Verification items for the finished model (mm, model axes). A direction names the side the tool comes from. Give positions to 0.01 mm unless a question says otherwise; leave off trailing zeros. Order: outer loops, then holes, each group sorted by start corner. A loop starts at its lowest first (then second) coordinate and runs counter-clockwise, first axis right, second up. Notation, with made-up numbers: (56, 54) - (96, 54) arc R30 cw to (96, 83) - close; hole circle Ø7 at (33.5, 66). An arc over 180 degrees is marked (long way). Answer as a JSON object with one key per item and string values.
Autodesk Inventor part; units mm, degrees
ref_plane "YZ Plane" through (0, 0, 0) normal (1, 0, 0) x (0, 1, 0)
ref_plane "XZ Plane" through (0, 0, 0) normal (0, 1, 0) x (-1, 0, 0)
ref_plane "XY Plane" through (0, 0, 0) normal (0, 0, 1) x (1, 0, 0)
sketch "スケッチ1" plane through (0, 0, 0) normal (1, 0, 0) x (0, 1, 0)
  line L0 (-20, 60) -> (20, 60)
  line L1 (20, 60) -> (20, -60)
  line L2 (20, -60) -> (-20, -60)
  line L3 (-20, -60) -> (-20, 60)
  point P0 (0, 0)
  dimension "d0" = 40
  dimension "d2" = 20
  dimension "d3" = 120
  dimension "d4" = 60
extrude "押し出し1" add sketch "スケッチ1" along normal blind 2
sketch "スケッチ2" plane through (2, 0, 0) normal (1, 0, 0) x (0, 0, -1)
  line L0 (-60, 20) -> (-60, -20)
  line L1 (-60, -20) -> (60, -20)
  line L2 (60, -20) -> (60, 20)
  line L3 (60, 20) -> (-60, 20)
  line L4 (-60, 6.6025) -> (-10, 20)
  line L5 (-40, -20) -> (-40, -8.0385)
  line L6 (-40, -8.0385) -> (-10, 0)
  line L7 (-10, 0) -> (60, 0)
  point P0 (0, 0)
  dimension "d7" = 20
  dimension "d8" = 20
  dimension "d9" = 70
  dimension "d10" = 15
  dimension "d11" = 70
extrude "押し出し2" cut sketch "スケッチ2" against normal blind 2 contours L4 L3 L2 L7 L6 L5 L1 L0 keep common part
sketch "スケッチ3" plane through (2, 0, 0) normal (1, 0, 0) x (0, 0, -1)
  line L0 (60, 0) -> (-10, 0)
  line L1 (60, 0) -> (60, 20)
  line L2 (-60, 6.6025) -> (-60, -20)
  line L3 (-60, -20) -> (-40, -20)
  line L4 (-54, -20) -> (-46, -20)
  line L5 (-46, -20) -> (-46, -16)
  line L6 (-54, -16) -> (-54, -20)
  line L7 (60, 14) -> (56, 14)
  line L8 (56, 6) -> (60, 6)
  line L9 (60, 6) -> (60, 14)
  arc A0 (-46, -16) -> (-54, -16) centre (-50, -16) ccw
  arc A1 (56, 14) -> (56, 6) centre (56, 10) ccw
  point P0 (0, 0)
  dimension "d14" = 8
  dimension "d16" = 8
  dimension "d19" = 4
  dimension "d20" = 4
  dimension "d21" = 10
  dimension "d22" = 4
  dimension "d23" = 4
  dimension "d24" = 10
  dimension "d26" = 4
  dimension "d27" = 4
extrude "押し出し3" cut sketch "スケッチ3" against normal blind 2
sketch "スケッチ4" plane through (2, 0, 0) normal (1, 0, 0) x (0, 0, -1)
  arc A0 (-46, -16) -> (-54, -16) centre (-50, -16) ccw
  arc A1 (56, 14) -> (56, 6) centre (56, 10) ccw
  circle A2 centre (-43, -16) radius 1
  circle A3 centre (56, 17) radius 1
  point P0 (0, 0)
  dimension "d30" = 2
  dimension "d32" = 7
  dimension "d33" = 0
  dimension "d34" = 7
  dimension "d35" = 0
hole "穴1" at (2, 17, -56) at (2, -16, 43) direction (-1, 0, 0) diameter 2 end through all
pattern_circular "円形状パターン1" count 5 over 180 about axis through (2, 10, -56) along (1, 0, 0) of "穴1"
pattern_circular "円形状パターン2" count 5 over 180 about axis through (2, -16, 50) along (1, 0, 0) of "穴1"
sketch "スケッチ5" plane through (2, 0, 0) normal (1, 0, 0) x (0, 0, -1)
  line L0 (60, 14) -> (60, 20)
  line L1 (60, 20) -> (-10, 20)
  circle A0 centre (-5, 17) radius 1
  circle A1 centre (5, 17) radius 1
  point P0 (0, 0)
  dimension "d49" = 10
  dimension "d51" = 3
  dimension "d52" = 3
  dimension "d53" = 2
  dimension "d54" = 55
hole "穴2" at (2, 17, -5) at (2, 17, 5) direction (-1, 0, 0) diameter 1.5 end through all
sketch "スケッチ6" plane through (2, 0, 0) normal (1, 0, 0) x (0, 0, -1)
  circle A0 centre (5, 17) radius 0.75
  circle A1 centre (-5, 17) radius 0.75
  circle A2 centre (-57, -16) radius 1
  circle A3 centre (-54.9497, -11.0503) radius 1
  circle A4 centre (-50, -9) radius 1
  circle A5 centre (-45.0503, -11.0503) radius 1
  circle A6 centre (56, 3) radius 1
  circle A7 centre (51.0503, 5.0503) radius 1
  circle A8 centre (49, 10) radius 1
  circle A9 centre (51.0503, 14.9497) radius 1
  circle A10 centre (56, 17) radius 1
  circle A11 centre (-43, -16) radius 1
  line L0 (56, 14) -> (60, 14)
  line L1 (60, 14) -> (60, 20)
  line L2 (60, 20) -> (-10, 20)
  line L3 (-60, 6.6025) -> (-10, 20)
  line L4 (-60, 6.6025) -> (-60, -20)
  line L5 (-60, -20) -> (-54, -20)
  line L6 (-54, -20) -> (-54, -16)
  arc A12 (-46, -16) -> (-54, -16) centre (-50, -16) ccw
  line L7 (-46, -16) -> (-46, -20)
  line L8 (-46, -20) -> (-40, -20)
  line L9 (-40, -8.0385) -> (-40, -20)
  line L10 (-10, 0) -> (-40, -8.0385)
  line L11 (60, 0) -> (-10, 0)
  line L12 (60, 0) -> (60, 6)
  line L13 (60, 6) -> (56, 6)
  arc A13 (56, 14) -> (56, 6) centre (56, 10) ccw
  arc A14 (-40.8348, -20) -> (-40, -16) centre (-50, -16) ccw
  arc A15 (-60, -16) -> (-59.1652, -20) centre (-50, -16) ccw
  arc A16 (60, 19.1652) -> (56, 20) centre (56, 10) ccw
  arc A17 (56, 0) -> (60, 0.8348) centre (56, 10) ccw
  point P0 (0, 0)
  dimension "d64" = 10
extrude "押し出し4" cut sketch "スケッチ6" against normal blind 2 contours A13 L13 L12 A17 L11 L10 L9 A14 L8 L7 A12 L6 L5 A15 L4 L3 L2 A16 L1 L0 keep common part
properties part number "Leg_Link_Flame" material "アルミニウム 6061"
(1) Material ranges on line 1 along Z through (x, y) = (1.5, -16); line 2 along Y through (x, z) = (0.5, -56); line 3 along Z through (x, y) = (1.1, 5), recorded low to high. Write a range as [from, to].
Computed values:
{"line 1": "z = [40, 42], [44, 46], [54, 56], [58, 60]", "line 2": "y = [0, 2], [4, 6], [14, 16], [18, 20]", "line 3": "z = [-60, -52.05], [-50.05, 60]"}
(2) Section check B-B (z = 32). Record the cut outline in (x, y), then the cut area to 3 significant figures.
Computed values:
{"outline": "(0, -5.89) - (2, -5.89) - (2, 14.11) - (0, 14.11) - close", "area": "40.0 mm²"}
(3) Access from +Z, -Z, +X, -X, +Y, -Y to the whole of each face (thin tool, end or side, straight path). Record for faces 1 (the flat face through (1, -18, 54)), 2 (the flat face through (1, 0, -23)), 3 (the flat face through (1, 17, -60)).
Computed values:
{"face 1": "+X, -X, -Y", "face 2": "-Z, +X, -X, -Y", "face 3": "-Z, +X, -X, +Y, -Y"}
(4) Gauge pin test, flat ends, axial feed: pin 1 Ø0.6 at (x, y) = (1.5, -18) entering from -Z; pin 2 Ø1.6 at (y, z) = (-16, 43) entering from -X; pin 3 Ø0.6 at (x, z) = (1.5, -57.5) entering from -Y; pin 4 Ø1 at (x, z) = (1, -23.5) entering from -Y. Record the tip position at first contact, or that the pin passes through.
Computed values:
{"pin 1": "stops at z = 40.15", "pin 2": "passes through", "pin 3": "stops at y = 0.07", "pin 4": "stops at y = 0"}
(5) Section check A-A (x = 0.85). Count the separate pieces of the cut face and the enclosed holes in it, then the cut area to 3 significant figures.
Computed values:
{"separate pieces": "1", "enclosed holes": "12", "area": "2,430 mm²"}
(6) Release check for a two-part mould opening along Z. For faces 4 (the flat face through (1, 6, -58)), 5 (the flat face through (1, -18, 46)), 6 (the flat face through (1, -5, 60)) record: pulls with the +Z half, pulls with the -Z half, needs draft (parallel to the pull), parting line crosses it, or undercut.
Computed values:
{"face 4": "needs draft", "face 5": "undercut", "face 6": "pulls with the +Z half"}
